```python
from build123d import *

# Parameters (mm, degrees)
F2_DEPTH = 6
F0_R     = 0.7500112
F0_R_2   = 0.7430174238
F3_DEPTH = 25.4


# Not quite as in the source:
# - ends of sketch curves that miss each other by under 0.0002 mm in the source are joined


with BuildPart() as f2:
    # F1 (on face) → F2 (new body)
    with BuildSketch(Plane.XZ):
        with BuildLine():
            Line((239.9250705835, 222.0849408719), (251.1754686974, 210.6445925623))
            ThreePointArc((251.1754686974, 210.6445925623), (252.1467535933, 209.9867437177), (253.2968294671, 209.755476289))
            Line((253.2968294671, 209.755476289), (254.8801768619, 209.755476289))
            ThreePointArc((254.8801768619, 209.755476289), (256.983999836, 210.6269082977), (257.8554318447, 212.7307312719))
            Line((257.8554318447, 212.7307312719), (257.8554318447, 243.475032761))
            ThreePointArc((257.8554318447, 243.475032761), (256.983999836, 245.5788557351), (254.8801768619, 246.4502877439))
            Line((254.8801768619, 246.4502877439), (-254.8801768619, 246.4502877439))
            ThreePointArc((-254.8801768619, 246.4502877439), (-256.983999836, 245.5788557351), (-257.8554318447, 243.475032761))
            Line((-257.8554318447, 243.475032761), (-257.8554318447, 212.7307312719))
            ThreePointArc((-257.8554318447, 212.7307312719), (-256.983999836, 210.6269082977), (-254.8801768619, 209.755476289))
            Line((-254.8801768619, 209.755476289), (-226.1193786946, 209.755476289))
            ThreePointArc((-226.1193786946, 209.755476289), (-224.0155557204, 208.8840442803), (-223.1441237117, 206.7802213062))
            Line((-223.1441237117, 206.7802213062), (-223.1441237117, -241.4915294391))
            Line((-223.1441237117, -241.4915294391), (-218.185365407, -246.4502877439))
            Line((-218.185365407, -246.4502877439), (218.185365407, -246.4502877439))
            Line((218.185365407, -246.4502877439), (223.1441237117, -241.4915294391))
            Line((223.1441237117, -241.4915294391), (223.1441237117, 208.5084705609))
            ThreePointArc((223.1441237117, 208.5084705609), (223.375391006, 209.658546114), (224.0332399627, 210.6298303616))
            Line((224.0332399627, 210.6298303616), (235.7175720959, 222.1201619404))
            ThreePointArc((235.7175720959, 222.1201619404), (237.8286155716, 222.9739529007), (239.9250705835, 222.0849408719))
        make_face()
        Polygon((72.2957914, 0), (36.1479084, -62.6100094), (-36.1479084, -62.6100094), (-72.2957914, 0), (-36.1479084, 62.6100094), (36.1479084, 62.6100094), align=None, mode=Mode.SUBTRACT)
    extrude(amount=F2_DEPTH)

    # F0 (on Front) → F3 (join)
    with BuildSketch(Plane.XZ):
        Polygon((36.1479084, -62.6100094), (72.2957914, 0), (36.1479084, 62.6100094), (-36.1479084, 62.6100094), (-72.2957914, 0), (-36.1479084, -62.6100094), align=None)
        with Locations((-34.993199, -60.609988)):
            Circle(F0_R, mode=Mode.SUBTRACT)
        with Locations((34.993199, -60.609988)):
            Circle(F0_R, mode=Mode.SUBTRACT)
        with Locations((-69.986398, 0)):
            Circle(F0_R, mode=Mode.SUBTRACT)
        with Locations((-34.993199, 60.609988)):
            Circle(F0_R, mode=Mode.SUBTRACT)
        with Locations((69.995796, 0)):
            Circle(F0_R_2, mode=Mode.SUBTRACT)
        with Locations((34.993199, 60.609988)):
            Circle(F0_R, mode=Mode.SUBTRACT)
        Polygon((72.47959348, -0.1061088931), (36.3364219227, -62.7188382077), (72.4890757311, -125.3261121412), (144.7848756936, -125.3206127679), (180.9280472508, -62.7078834532), (144.7753934424, -0.1006095197), align=None)
        with Locations((73.6436387774, -123.3260062512)):
            Circle(F0_R, mode=Mode.SUBTRACT)
        with Locations((143.6300274078, -123.3207069419)):
            Circle(F0_R, mode=Mode.SUBTRACT)
        with Locations((38.6458459563, -62.7186601398)):
            Circle(F0_R, mode=Mode.SUBTRACT)
        with Locations((73.6297421488, -2.0978761685)):
            Circle(F0_R_2, mode=Mode.SUBTRACT)
        with Locations((178.6186232172, -62.7080615211)):
            Circle(F0_R, mode=Mode.SUBTRACT)
        with Locations((143.6208303961, -2.1007154097)):
            Circle(F0_R, mode=Mode.SUBTRACT)
        Polygon((36.1478997424, -62.8259687739), (-36.1479168252, -62.8201722222), (-72.3008196697, -125.4272831471), (-36.1579567466, -188.0401906197), (36.1378598211, -188.0459871714), (72.2907626655, -125.4388762464), align=None)
        with Locations((-35.0030869921, -186.0402618087)):
            Circle(F0_R, mode=Mode.SUBTRACT)
        with Locations((-69.9914262771, -125.4274683102)):
            Circle(F0_R, mode=Mode.SUBTRACT)
        with Locations((-34.9933677872, -64.8202861983)):
            Circle(F0_R, mode=Mode.SUBTRACT)
        with Locations((34.983310783, -186.0458731952)):
            Circle(F0_R, mode=Mode.SUBTRACT)
        with Locations((69.9907672729, -125.4386918368)):
            Circle(F0_R_2, mode=Mode.SUBTRACT)
        with Locations((34.9930299879, -64.8258975849)):
            Circle(F0_R, mode=Mode.SUBTRACT)
        Polygon((-36.3200081195, -62.7093545109), (-72.4588066668, -0.0941010816), (-144.7546060688, -0.0835525132), (-180.91163233, -62.6883013644), (-144.7728337827, -125.3035547937), (-72.4770343807, -125.3141033621), align=None)
        with Locations((-143.6225460101, -123.3118678504)):
            Circle(F0_R_2, mode=Mode.SUBTRACT)
        with Locations((-73.6314577352, -123.3139168414)):
            Circle(F0_R, mode=Mode.SUBTRACT)
        with Locations((-178.6022083144, -62.6886407243)):
            Circle(F0_R, mode=Mode.SUBTRACT)
        with Locations((-143.6001827143, -2.0837390339)):
            Circle(F0_R, mode=Mode.SUBTRACT)
        with Locations((-38.6294321351, -62.709015151)):
            Circle(F0_R, mode=Mode.SUBTRACT)
        with Locations((-73.6137946247, -2.0939262472)):
            Circle(F0_R, mode=Mode.SUBTRACT)
        Polygon((-72.4855936704, 0.1095682125), (-36.3446929989, 62.7236083401), (-72.4996174478, 125.3295710344), (-144.7954171632, 125.3214496097), (-180.9363178347, 62.7074094821), (-144.7813933858, 0.1014467878), align=None)
        with Locations((-143.6269028809, 2.1015945506)):
            Circle(F0_R, mode=Mode.SUBTRACT)
        with Locations((-178.626893809, 62.707671309)):
            Circle(F0_R, mode=Mode.SUBTRACT)
        with Locations((-73.6405144887, 2.1094321527)):
            Circle(F0_R, mode=Mode.SUBTRACT)
        with Locations((-38.6541170246, 62.7233465131)):
            Circle(F0_R, mode=Mode.SUBTRACT)
        with Locations((-143.645196257, 123.3297240496)):
            Circle(F0_R_2, mode=Mode.SUBTRACT)
        with Locations((-73.6541079527, 123.3294232716)):
            Circle(F0_R, mode=Mode.SUBTRACT)
        Polygon((-36.1479091406, 62.8225415071), (36.1479076577, 62.8230453272), (72.2953543359, 125.4333066355), (36.1470350159, 188.0430641241), (-36.1487817824, 188.0425603041), (-72.2962284606, 125.4322989958), align=None)
        with Locations((-34.9932136785, 64.8225709541)):
            Circle(F0_R, mode=Mode.SUBTRACT)
        with Locations((-69.9868350606, 125.4323150896)):
            Circle(F0_R, mode=Mode.SUBTRACT)
        with Locations((-34.9940584445, 186.0425469512)):
            Circle(F0_R, mode=Mode.SUBTRACT)
        with Locations((34.9931843198, 64.8230586801)):
            Circle(F0_R, mode=Mode.SUBTRACT)
        with Locations((69.995358936, 125.4332906071)):
            Circle(F0_R_2, mode=Mode.SUBTRACT)
        with Locations((34.9923395538, 186.0430346772)):
            Circle(F0_R, mode=Mode.SUBTRACT)
        Polygon((36.3247836852, 62.71214389), (72.4809283845, 0.1069051082), (144.7767279344, 0.1163860718), (180.9164081792, 62.7311498147), (144.7602634799, 125.3363885966), (72.46446393, 125.3269076329), align=None)
        with Locations((73.6306643166, 2.098910662)):
            Circle(F0_R_2, mode=Mode.SUBTRACT)
        with Locations((38.6342077061, 62.7124443555)):
            Circle(F0_R, mode=Mode.SUBTRACT)
        with Locations((143.6217504731, 2.116252683)):
            Circle(F0_R, mode=Mode.SUBTRACT)
        with Locations((178.6069841582, 62.7308493493)):
            Circle(F0_R, mode=Mode.SUBTRACT)
        with Locations((73.6194413913, 123.3270410217)):
            Circle(F0_R, mode=Mode.SUBTRACT)
        with Locations((143.6058296174, 123.3362435186)):
            Circle(F0_R, mode=Mode.SUBTRACT)
    extrude(amount=F3_DEPTH)


solid = f2.part
```
Input: part model. Units: mm. Frame: model coordinates. A direction names the side the tool comes from. Round coordinates to 2 decimals unless told otherwise and drop trailing zeros. Loops run counter-clockwise (first coordinate to the right, second up) from the corner with the lowest first, then second, coordinate; pieces in that order, holes last.
1) Pull-direction query (Z, two-part tool) for faces 4 (the flat face through (-54.136, -15.564, -31.84)), 5 (the flat face through (-53.969, -15.564, 157.176)), 6 (the flat face through (-163.095, -15.564, -93.558)); classes: released by +Z, released by -Z, zero draft, split by the parting line, or undercut.
Ans:
face 4: undercut
face 5: released by +Z
face 6: released by -Z
2) Material intervals for line 1 (X direction, y = -20.5, z = 117.5); line 2 (X direction, y = -9.5, z = 47); line 3 (Z direction, x = 113, y = -12), sorted ascending.
Ans:
line 1: x = -149.31 to -67.98, -67.72 to 67.72, 67.95 to 149.29
line 2: x = -171.87 to -45.42, -45.16 to 45.16, 45.4 to 171.84
line 3: z = -125.32 to -0.1, 0.11 to 125.33
3) Set-up query: faces 1 (the flat face through (163.09, -15.56, 93.6)), 2 (the flat face through (-61, -6, 168)), 3 (the flat face through (-163.11, -15.56, 31.84)). Return all of +Z, -Z, +X, -X, +Y, -Y with unobstructed straight access to the full face (end or side cutting, diameter ignored); none if empty.
Ans:
face 1: +Z, +X, -Y
face 2: -Y
face 3: -X, -Y
4) Section query D-D on z = 52.5. Return the cut outline in (x, y).
Ans:
outline: (-223.14, -6) - (-175.04, -6) - (-175.04, -25.4) - (-42.25, -25.4) - (-42.25, -6) - (-41.98, -6) - (-41.98, -25.4) - (41.98, -25.4) - (41.98, -6) - (42.22, -6) - (42.22, -25.4) - (175.01, -25.4) - (175.01, -6) - (223.14, -6) - (223.14, 0) - (-223.14, 0) - close
5) Pin query (flat end, axial travel): pin 1 (1.3 mm diameter, centred on x = -143.65, z = 123.33, fed in from -Y); pin 2 (1.2 mm diameter, centred on x = -144, z = 2, fed in from -Y); pin 3 (1.2 mm diameter, centred on x = -69.99, z = 0, fed in from +Y); pin 4 (4 mm diameter, centred on x = 106.5, y = -15.5, fed in from -Z). Return the tip coordinate at first contact, or that it passes through.
Ans:
pin 1: stops at y = -6
pin 2: stops at y = -25.4
pin 3: passes through
pin 4: stops at z = -125.32
6) Section query C-C on x = 48. Return the cut outline in (y, z), plus the area to 3 significant figures.
Ans:
outline: (-25.4, -167.5) - (-6, -167.5) - (-6, -246.45) - (0, -246.45) - (0, 246.45) - (-6, 246.45) - (-6, 167.51) - (-25.4, 167.51) - (-25.4, 83.35) - (-6, 83.35) - (-6, 82.94) - (-25.4, 82.94) - (-25.4, 42.5) - (-6, 42.5) - (-6, 42.08) - (-25.4, 42.08) - (-25.4, -42.08) - (-6, -42.08) - (-6, -42.51) - (-25.4, -42.51) - (-25.4, -82.92) - (-6, -82.92) - (-6, -83.36) - (-25.4, -83.36) - close
area: 9,420 mm2
7) Section query A-A on z = -110.5. Return the cut outline in (x, y), plus the area to 3 significant figures.
Ans:
outline: (-223.14, -6) - (-153.32, -6) - (-153.32, -25.4) - (-63.92, -25.4) - (-63.92, -6) - (-63.68, -6) - (-63.68, -25.4) - (63.67, -25.4) - (63.67, -6) - (63.93, -6) - (63.93, -25.4) - (153.34, -25.4) - (153.34, -6) - (223.14, -6) - (223.14, 0) - (-223.14, 0) - close
area: 8,620 mm2
8) Section query B-B on y = -18. Count the separate pieces of the cut face and the enclosed holes in it, plus the area to 3 significant figures.
Ans:
separate pieces: 7
enclosed holes: 42
area: 95,000 mm2
